Can you work these out from the model? Positions are in its coordinate system, mm. A direction names the side the tool comes from. Round coordinates to 2 decimals unless told otherwise and drop trailing zeros. Order: outer loops, then holes, each group sorted by start corner. A loop starts at its lowest first (then second) coordinate and runs counter-clockwise, first axis right, second up. Notation, with made-up numbers: M 4,42.25 L 39,42.25 A17 ccw 39,74.25 Z; hole C 37,38 d3. An arc over 180 degrees is marked long. One line per question, with ' | ' between items.
```python
from build123d import *

# Parameters (mm, degrees)
BOSS_EXTRUDE1_DEPTH = 3
BOSS_EXTRUDE2_DEPTH = 26.999994
CHAMFER1_SIZE       = 3
CUT_EXTRUDE1_DEPTH  = 4.999994
SKETCH4_3_R         = 7.75
CUT_EXTRUDE2_DEPTH  = 4
SKETCH7_R           = 2.55
BOSS_EXTRUDE5_DEPTH = 5


with BuildPart() as part:
    # Sketch2 → Boss-Extrude1 (new body)
    with BuildSketch(Plane.XY.offset(26.999993563)):
        with BuildLine():
            Line((-48.107762328, -39.75057759), (11.056310458, -14.145221365))
            ThreePointArc((11.056310458, -14.145221365), (37.914072471, -25.999413947), (24.018554683, -51.86011478))
            Line((24.018554683, -51.86011478), (-38.38607916, -68.036747651))
            ThreePointArc((-38.38607916, -68.036747651), (-56.335559182, -58.392101106), (-48.107762328, -39.75057759))
        make_face()
    extrude(amount=BOSS_EXTRUDE1_DEPTH)

    # Sketch3 → Boss-Extrude2 (add)
    with BuildSketch(Plane(origin=(0, 0, 26.999993563), x_dir=(-1, 0, 0), z_dir=(0, 0, -1))):
        with BuildLine():
            Line((48.107762328, -39.75057759), (-11.056310458, -14.145221365))
            ThreePointArc((-11.056310458, -14.145221365), (-37.914072471, -25.999413947), (-24.018554683, -51.86011478))
            Line((-24.018554683, -51.86011478), (38.38607916, -68.036747651))
            ThreePointArc((38.38607916, -68.036747651), (56.335559182, -58.392101106), (48.107762328, -39.75057759))
        make_face()
        with BuildLine():
            Line((46.916209863, -42.503794385), (-12.247862924, -16.89843816))
            ThreePointArc((-12.247862924, -16.89843816), (-35.076960635, -26.974501855), (-23.265770515, -48.956097563))
            Line((-23.265770515, -48.956097563), (39.138863328, -65.132730434))
            ThreePointArc((39.138863328, -65.132730434), (53.498447346, -57.417013198), (46.916209863, -42.503794385))
        make_face(mode=Mode.SUBTRACT)
    extrude(amount=BOSS_EXTRUDE2_DEPTH)

    # Chamfer1
    chamfer1_edges = [part.edges().sort_by_distance(p)[0] for p in [
        (37.914072471, -25.999413947, 29.999993563),
        (-18.525725935, -26.947899478, 29.999993563),
        (-53.498447346, -57.417013198, 26.999993563),
        (-17.334173469, -29.701116273, 26.999993563),
        (35.076960635, -26.974501855, 26.999993563),
        (-7.936546407, -57.044413998, 26.999993563),
        (-56.335559182, -58.392101106, 29.999993563),
        (-7.183762238, -59.948431215, 29.999993563),
    ]]
    chamfer(chamfer1_edges, length=CHAMFER1_SIZE)

    # Sketch4 → Cut-Extrude1 (cut)
    with BuildSketch(Plane.XY.offset(4.999993563)):
        Polygon((-63.676072098, -10.5), (2, -10.5), (2, -39.366661566), (-18, -39.366661566), (-18, -71.666661566), (-63.676072098, -71.666661566), align=None)
    extrude(amount=-CUT_EXTRUDE1_DEPTH, mode=Mode.SUBTRACT)

    # Sketch4<3> → Cut-Extrude2 (cut)
    with BuildSketch(Plane.XY.offset(4.999993563)):
        with Locations((-10, -25.866661566)):
            Circle(SKETCH4_3_R)
    extrude(amount=CUT_EXTRUDE2_DEPTH, mode=Mode.SUBTRACT)

    # Sketch7 → Boss-Extrude5 (add)
    with BuildSketch(Plane(origin=(0, 0, 0), x_dir=(-1, 0, 0), z_dir=(0, 0, -1))):
        with BuildLine():
            Line((-8.999993562, -55.753251147), (-8.999993562, -70))
            ThreePointArc((-8.999993562, -70), (-10.464459657, -73.535533906), (-13.999993562, -75))
            Line((-13.999993562, -75), (-23.999993562, -75))
            ThreePointArc((-23.999993562, -75), (-27.535527468, -73.535533906), (-28.999993562, -70))
            Line((-28.999993562, -70), (-28.999993562, -49.820508076))
            ThreePointArc((-28.999993562, -49.820508076), (-26.578205318, -51.008665716), (-24.018554683, -51.86011478))
            Line((-24.018554683, -51.86011478), (-8.999993562, -55.753251147))
        make_face()
        with Locations((-18.999993562, -65)):
            Circle(SKETCH7_R, mode=Mode.SUBTRACT)
    extrude(amount=-BOSS_EXTRUDE5_DEPTH)


solid = part.part
```
(1) Please list where these lines run through material, in increasing order: probe 1 along Z at (x, y) = (-3, -50.5); probe 2 along Y at (x, z) = (2, 8.75); probe 3 along Y at (x, z) = (-19, 13.5). Write a range as [from, to].
Final values:
probe 1: [27, 30] | probe 2: [-57.57, -54.47], [-21.33, -18.06] | probe 3: [-63.01, -59.91], [-30.42, -27.15]
(2) If we section it at C-C on y = -32.5: Please give me the cut outline in (x, z).
Final values:
outline: M -31.35,5 L -23.8,5 L -23.8,24 L -16.25,27 L 33,27 L 36,24 L 36,0 L 39,0 L 39,27 L 36,30 L -23.8,30 L -31.35,27 Z
(3) Will these pins go through, and if not, where does the flat tip stop? pin 1 Ø2.5 at (x, y) = (-14, -25.5) entering from -Z; pin 2 Ø6 at (x, z) = (9.5, 26) entering from -Y; pin 3 Ø2.5 at (y, z) = (-61.5, 3) entering from -X.
Final values:
pin 1: z = 9 | pin 2: y = -56.4 | pin 3: x = -18
(4) If we section it at A-A on z = 17: Please give me the cut outline in (x, y).
Final values:
outline: M -48.11,-39.75 A15 ccw -38.39,-68.04 L 24.02,-51.86 A20 ccw long 11.06,-14.15 Z; hole M -46.92,-42.5 A12 ccw -39.14,-65.13 L 23.27,-48.96 A17 ccw long 12.25,-16.9 Z
(5) If we section it at B-B on x = -33: Please give me the cut outline in (y, z), plus the area to 3 significant figures.
Final values:
outline: M -66.64,5 L -63.54,5 L -63.54,24 L -60.44,27 L -39.75,27 L -36.48,24 L -36.48,5 L -33.21,5 L -33.21,27 L -36.48,30 L -63.54,30 L -66.64,27 Z | area: 240 mm^2
(6) On a 3-axis mill with a long thin cutter (end or side, diameter ignored), from which of +Z, -Z, +X, -X, +Y, -Y can I reach the whole of each face in a straight line? I mean faces 5 (the flat face through (2, -20, 3)), 6 (the cylindrical face through (-17.43, -28.07, 6.97)), 7 (the flat face through (-7.5, -56.93, 12.17)), 8 (the cylindrical face through (-3.29, -21.99, 6.97)), 9 (the flat face through (-18.352, -28.484, 28.479)). Say none if no direction works.
Final values:
face 5: -Z, -X, +Y | face 6: -Z, +Y | face 7: -Z | face 8: -Z, -X | face 9: +Z, -X, +Y
(7) Thinking about a two-plate mould opening in Y: for faces 1 (the flat face through (0, -21, 5)), 2 (the cylindrical face through (37.759, -25.565, 13.689)), 3 (the cylindrical face through (27, -74, 2)), 4 (the cylindrical face through (20.9, -63.3, 2.5)), which applies, released by +Y, released by -Y, zero draft, split by the parting line, or undercut?
Final values:
face 1: zero draft | face 2: split by the parting line | face 3: released by -Y | face 4: undercut
